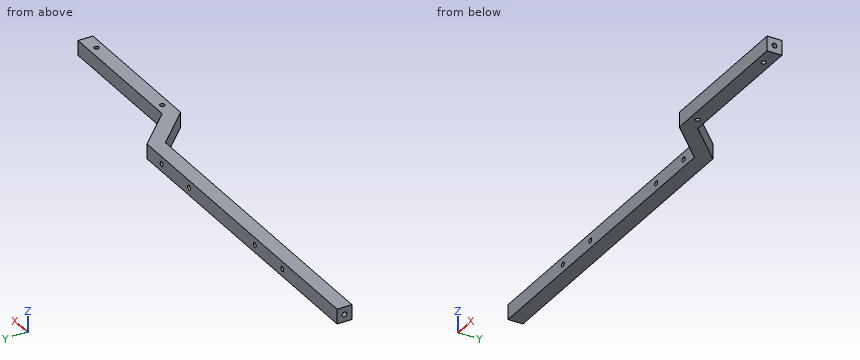
```python
from build123d import *

# Parameters (mm, degrees)
SKETCH2_W           = 8
SKETCH2_H           = 130
BOSS_EXTRUDE1_DEPTH = 8
CUT_EXTRUDE1_REACH  = 67.977
SKETCH4_R           = 1.3
BOSS_EXTRUDE2_DEPTH = 8
SKETCH8_R           = 1.3
CUT_EXTRUDE3_DEPTH  = 10
CUT_EXTRUDE4_REACH  = 169.55
SKETCH9_R           = 1.3
SKETCH10_W          = 40
SKETCH10_H          = 8
BOSS_EXTRUDE3_DEPTH = 8
SKETCH11_R          = 1.3
CUT_EXTRUDE5_DEPTH  = 10


with BuildPart() as part:
    # Sketch2 → Boss-Extrude1 (new body)
    with BuildSketch(Plane(origin=(0, 0, 0), x_dir=(0, 1, 0), z_dir=(0, 0, 1))):
        with Locations((-4, 0)):
            Rectangle(SKETCH2_W, SKETCH2_H)
    extrude(amount=BOSS_EXTRUDE1_DEPTH)

    # Sketch4 → Cut-Extrude1 (cut, up to next)
    with BuildSketch(Plane(origin=(0, 0, 0), x_dir=(-1, 0, 0), z_dir=(0, 1, 0)), mode=Mode.PRIVATE) as cut_extrude1_sk1:
        with Locations((-55, 4)):
            Circle(SKETCH4_R)
    cut_extrude1_tool1 = extrude(cut_extrude1_sk1.sketch, amount=-CUT_EXTRUDE1_REACH, mode=Mode.PRIVATE) & part.part
    # Sketch4 → Cut-Extrude1 (cut, up to next)
    with BuildSketch(Plane(origin=(0, 0, 0), x_dir=(-1, 0, 0), z_dir=(0, 1, 0)), mode=Mode.PRIVATE) as cut_extrude1_sk2:
        with Locations((-30, 4)):
            Circle(SKETCH4_R)
    cut_extrude1_tool2 = extrude(cut_extrude1_sk2.sketch, amount=-CUT_EXTRUDE1_REACH, mode=Mode.PRIVATE) & part.part
    # Sketch4 → Cut-Extrude1 (cut, up to next)
    with BuildSketch(Plane(origin=(0, 0, 0), x_dir=(-1, 0, 0), z_dir=(0, 1, 0)), mode=Mode.PRIVATE) as cut_extrude1_sk3:
        with Locations((30, 4)):
            Circle(SKETCH4_R)
    cut_extrude1_tool3 = extrude(cut_extrude1_sk3.sketch, amount=-CUT_EXTRUDE1_REACH, mode=Mode.PRIVATE) & part.part
    # Sketch4 → Cut-Extrude1 (cut, up to next)
    with BuildSketch(Plane(origin=(0, 0, 0), x_dir=(-1, 0, 0), z_dir=(0, 1, 0)), mode=Mode.PRIVATE) as cut_extrude1_sk4:
        with Locations((55, 4)):
            Circle(SKETCH4_R)
    cut_extrude1_tool4 = extrude(cut_extrude1_sk4.sketch, amount=-CUT_EXTRUDE1_REACH, mode=Mode.PRIVATE) & part.part
    add(cut_extrude1_tool1.solids().sort_by_distance((55, 0, 4))[0], mode=Mode.SUBTRACT)
    add(cut_extrude1_tool2.solids().sort_by_distance((30, 0, 4))[0], mode=Mode.SUBTRACT)
    add(cut_extrude1_tool3.solids().sort_by_distance((-30, 0, 4))[0], mode=Mode.SUBTRACT)
    add(cut_extrude1_tool4.solids().sort_by_distance((-55, 0, 4))[0], mode=Mode.SUBTRACT)

    # Sketch7 → Boss-Extrude2 (add)
    with BuildSketch(Plane(origin=(0, 0, 0), x_dir=(1, 0, 0), z_dir=(0, 0, -1))):
        Polygon((65, 8), (85, 28), (165, 28), (165, 20), (88.313708499, 20), (68.313708499, 0), (65, 0), align=None)
    extrude(amount=-BOSS_EXTRUDE2_DEPTH)

    # Sketch8 → Cut-Extrude3 (cut)
    with BuildSketch(Plane.YZ.offset(165)):
        with Locations(Location((-24, 4, 0), (0, 0, 270))):
            Circle(SKETCH8_R)
    extrude(amount=-CUT_EXTRUDE3_DEPTH, mode=Mode.SUBTRACT)

    # Sketch9 → Cut-Extrude4 (cut, up to next)
    with BuildSketch(Plane(origin=(0, 0, 0), x_dir=(1, 0, 0), z_dir=(0, 0, -1)), mode=Mode.PRIVATE) as cut_extrude4_sk1:
        with Locations(Location((95, 24, 0), (0, 0, 180))):
            Circle(SKETCH9_R)
    cut_extrude4_tool1 = extrude(cut_extrude4_sk1.sketch, amount=-CUT_EXTRUDE4_REACH, mode=Mode.PRIVATE) & part.part
    # Sketch9 → Cut-Extrude4 (cut, up to next)
    with BuildSketch(Plane(origin=(0, 0, 0), x_dir=(1, 0, 0), z_dir=(0, 0, -1)), mode=Mode.PRIVATE) as cut_extrude4_sk2:
        with Locations((155, 24)):
            Circle(SKETCH9_R)
    cut_extrude4_tool2 = extrude(cut_extrude4_sk2.sketch, amount=-CUT_EXTRUDE4_REACH, mode=Mode.PRIVATE) & part.part
    add(cut_extrude4_tool1.solids().sort_by_distance((95, -24, 0))[0], mode=Mode.SUBTRACT)
    add(cut_extrude4_tool2.solids().sort_by_distance((155, -24, 0))[0], mode=Mode.SUBTRACT)

    # Sketch10 → Boss-Extrude3 (add)
    with BuildSketch(Plane.XY.offset(8)):
        with Locations((-85, -4)):
            Rectangle(SKETCH10_W, SKETCH10_H)
    extrude(amount=-BOSS_EXTRUDE3_DEPTH)

    # Sketch11 → Cut-Extrude5 (cut)
    with BuildSketch(Plane(origin=(-105, 0, 0), x_dir=(0, -1, 0), z_dir=(-1, 0, 0))):
        with Locations(Location((4, 4, 0), (0, 0, 90))):
            Circle(SKETCH11_R)
    extrude(amount=-CUT_EXTRUDE5_DEPTH, mode=Mode.SUBTRACT)


solid = part.part
```
Source: CAD feature listing. Evaluate the final solid. Frame: model axes, mm. Give positions to 0.01 mm unless a question says otherwise; leave off trailing zeros. Write each loop counter-clockwise with the first axis right and the second up, starting at its lowest first coordinate (ties: lowest second). Pieces come first, ordered by that corner, then holes.
1. Section query A-A (x = -84.5). Return the cut outline in (y, z).
2. First-contact query: pin 1 (4 mm diameter, centred on y = -13, z = 3, fed in from -X); pin 2 (1.5 mm diameter, centred on y = -11.5, z = 7, fed in from +X); pin 3 (2 mm diameter, centred on y = -4, z = 4, fed in from -X). Flat tips, straight axial feed; report the tip coordinate or a pass-through.
3. Material intervals for line 1 along Y through (x, z) = (161.25, 4); line 2 along Z through (x, y) = (55, -6.5); line 3 along Y through (x, z) = (135.5, 3.5), sorted ascending.
4. Section query B-B (y = -12.5). Return the cut outline in (x, z).
Output values:
1. outline: (-8, 0) - (0, 0) - (0, 8) - (-8, 8) - close
2. pin 1: stops at x = 68
2. pin 2: stops at x = 80.56
2. pin 3: stops at x = -95
3. line 1: y = -28 to -25.3, -22.7 to -20
3. line 2: z = 0 to 2.7, 5.3 to 8
3. line 3: y = -28 to -20
4. outline: (69.5, 0) - (80.81, 0) - (80.81, 8) - (69.5, 8) - close
